Autodesk Inventor part; units mm, degrees
ref_plane "Work Plane1" through (0, 14, 0) normal (0, 1, 0) x (-1, 0, 0)
ref_plane "Work Plane2" through (0, 16, 0) normal (0, 1, 0) x (-1, 0, 0)
ref_plane "YZ Plane" through (0, 0, 0) normal (1, 0, 0) x (0, 1, 0)
sketch "Sketch1" plane through (0, 0, 0) normal (1, 0, 0) x (0, 1, 0)
  line L0 (0, 0) -> (14, 0)
  line L1 (14, 0) -> (14, -40)
  line L2 (14, -40) -> (14.5, -40)
  line L3 (14.5, -40) -> (14.5, -70)
  line L4 (14.5, -70) -> (15, -70)
  line L5 (15, -70) -> (15, -114.5)
  line L6 (15, -114.5) -> (16, -114.5)
  line L7 (16, -114.5) -> (16, -150.5)
  line L8 (16, -150.5) -> (21, -150.5)
  line L9 (21, -150.5) -> (21, -156.5)
  line L10 (21, -156.5) -> (15, -156.5)
  line L11 (15, -156.5) -> (15, -194)
  line L12 (0, -232.8) -> (0, 38.8)
  line L13 (15, -194) -> (0, -194)
  dimension "d0" = 40
  dimension "d1" = 14
  dimension "d2" = 30
  dimension "d3" = 14.5
  dimension "d4" = 15
  dimension "d5" = 44.5
  dimension "d9" = 16
  dimension "d10" = 21
  dimension "d11" = 6
  dimension "d12" = 37.5
  dimension "d14" = 36
  dimension "d24" = 15
revolve "Revolution1" add sketch "Sketch1" angle 360 about axis through (0, 0, -10) along (0, 0, 1)
chamfer "Chamfer1" distance 1 angle 45 2 edges at (0, -15, -194) (0, -14, 0)
fillet "Fillet1" radius 3 1 edges at (0, -15, -156.5)
fillet "Fillet2" radius 2 1 edges at (0, -16, -150.5)
fillet "Fillet3" radius 1 1 edges at (0, -15, -114.5)
fillet "Fillet4" radius 0.5 2 edges at (0, -14.5, -70) (0, -14, -40)
ref_plane "Work Plane1" through (0, 14, 0) normal (0, 1, 0) x (-1, 0, 0)
sketch "Sketch2" plane through (0, 14, 0) normal (0, 1, 0) x (-1, 0, 0)
  line L0 (0, -40.8) -> (0, 6.8)
  line L1 (0, -10) -> (0, -30) construction
  line L2 (-4, -10) -> (-4, -30)
  line L3 (4, -30) -> (4, -10)
  arc A0 (4, -10) -> (-4, -10) centre (0, -10) ccw
  arc A1 (-4, -30) -> (4, -30) centre (0, -30) ccw
  point P0 (0, 0)
  point P1 (0, -20)
  dimension "d26" = 10
  dimension "d27" = 8
  dimension "d28" = 20
extrude "Extrusion1" cut sketch "Sketch2" against normal blind 4
ref_plane "Work Plane2" through (0, 16, 0) normal (0, 1, 0) x (-1, 0, 0)
sketch "Sketch3" plane through (0, 16, 0) normal (0, 1, 0) x (-1, 0, 0)
  line L0 (0, -177) -> (0, 29.5)
  line L1 (0, -143.5) -> (0, -123.5) construction
  line L2 (4, -143.5) -> (4, -123.5)
  line L3 (-4, -123.5) -> (-4, -143.5)
  arc A0 (-4, -143.5) -> (4, -143.5) centre (0, -143.5) ccw
  arc A1 (4, -123.5) -> (-4, -123.5) centre (0, -123.5) ccw
  line L4 (-15, -113.5) -> (15, -113.5)
  line L5 (-16, -114.5) -> (16, -114.5)
  point P0 (0, 0)
  point P1 (0, -133.5)
  dimension "d32" = 8
  dimension "d34" = 9
  dimension "d35" = 20
extrude "Extrusion2" cut sketch "Sketch3" against normal blind 5
properties part number "Truc_2"
Check sheet for the modelled part. Datum: model origin and axes. Units: mm. A direction names the side the tool comes from. Round coordinates to 2 decimals unless told otherwise and drop trailing zeros. Loops run counter-clockwise (first coordinate to the right, second up) from the corner with the lowest first, then second, coordinate; pieces in that order, holes last. Notation, with made-up numbers: (59, 38) - (71, 38) arc R15 ccw to (71, 65) - close; hole circle Ø5 at (-25.75, 5). An arc over 180 degrees is marked (long way). Answer as CSV lines item,"result". Start each with the question number.
Item 1: Section check A-A (z = -140). Record the boundary of the cut face in (x, y).
Item 2: Set-up check for faces 4 (the cylindrical face through (-15.62, -3.47, -131.74)), 5 (the flat face through (0, 11, -133)), 6 (the flat face through (0, 0, -194)): record each of +Z, -Z, +X, -X, +Y, -Y from which the full face is reachable in a straight line by a thin tool's end or side.
Item 3: Release check for a two-part mould opening along Z. For faces 1 (the cylindrical face through (-12.864, 6.691, -54.957)), 2 (the cylindrical face through (-0.1, 13.5, -119.5)), 3 (the flat face through (0, 0, 0)) record: +Z half, -Z half, draft (parallel to the pull), parting line (faces both ways), or undercut.
Item 4: Section check B-B (z = -169.5). Record the boundary of the cut face in (x, y).
Item 5: Section check C-C (z = -14.5). Record the boundary of the cut face in (x, y).
Item 6: Scan lines: line 1 (Y direction, x = 10.5, z = -61); line 2 (X direction, y = 0.5, z = -68); line 3 (Z direction, x = 12.5, y = 15.5). Record each from-to range of solid material in increasing order. Write a range as [from, to].
Item 7: Depth check by flat-ended pin: P1, Ø5, axis at x = -13.5, y = 15.5, coming from the +Z side; P2, Ø3.5, axis at y = 12.5, z = -132.5, coming from the +X side; P3, Ø10, axis at x = 14.5, z = -99.5, coming from the -Y side; P4, Ø2, axis at x = -16, z = -28, coming from the +Y side. Enter the tip coordinate at first touch or a pass-through.
Report:
1,outline,"(-4, 11) - (-4, 15.49) arc R16 ccw (long way) to (4, 15.49) - (4, 11) - close"
2,face 4,"+Z"
2,face 5,"+Y"
2,face 6,"-Z, +X, -X, +Y, -Y"
3,face 1,"draft"
3,face 2,"undercut"
3,face 3,"+Z half"
4,outline,"circle Ø30 at (0, 0)"
5,outline,"(-4, 10) - (-4, 13.42) arc R14 ccw (long way) to (4, 13.42) - (4, 10) - close"
6,line 1,"y = [-10, 10]"
6,line 2,"x = [-14.49, 14.49]"
6,line 3,"z = [-156.5, -150.5]"
7,P1,"stops at z = -150.5"
7,P2,"stops at x = 11.85"
7,P3,"stops at y = -11.61"
7,P4,"passes through"
